Model file for the job. Use its own axes, mm. A direction names the side the tool comes from. Give positions to 0.01 mm unless a question says otherwise; leave off trailing zeros. Write each loop counter-clockwise with the first axis right and the second up, starting at its lowest first coordinate (ties: lowest second). Pieces come first, ordered by that corner, then holes. Notation, with made-up numbers: (-36, 86) - (-29, 86) arc R12 ccw to (-29, 100) - close; hole circle Ø6 at (46, 66.25). An arc over 180 degrees is marked (long way). Use a Markdown table: item, result. Add a question column.
```python
from build123d import *

# Parameters (mm, degrees)
F0_W      = 29
F0_H      = 16.5
F1_DEPTH  = 38.5
F2_SIZE   = 2
F3_SIZE   = 2
F4_SIZE   = 1
F5_W      = 25
F5_H      = 12.5
F6_DEPTH  = 34.25
F8_DEPTH  = 16.501
F9_W      = 12.5
F9_H      = 1
F10_DEPTH = 25
F11_W     = 7.54
F11_H     = 7.25
F11_R     = 1.1
F12_DEPTH = 4.35
F13_R     = 2
F14_DEPTH = 25
F15_W     = 5.538
F15_H     = 5.533
F17_W     = 5.538
F17_H     = 4.538


with BuildPart() as f1:
    # F0 (on Top) → F1 (new body)
    with BuildSketch(Plane.XY):
        with Locations((14.5, 8.25)):
            Rectangle(F0_W, F0_H)
    extrude(amount=F1_DEPTH)

    # F2
    f2_edges = [f1.edges().sort_by_distance(p)[0] for p in [
        (0, 0, 19.25),
        (0, 16.5, 19.25),
        (29, 0, 19.25),
        (29, 16.5, 19.25),
    ]]
    chamfer(f2_edges, length=F2_SIZE)

    # F3
    f3_edges = [f1.edges().sort_by_distance(p)[0] for p in [
        (0, 8.25, 0),
        (1, 15.5, 0),
        (1, 1, 0),
        (14.5, 16.5, 0),
        (14.5, 0, 0),
        (28, 15.5, 0),
        (28, 1, 0),
        (29, 8.25, 0),
    ]]
    chamfer(f3_edges, length=F3_SIZE)

    # F4
    f4_edges = [f1.edges().sort_by_distance(p)[0] for p in [
        (0, 8.25, 38.5),
        (1, 15.5, 38.5),
        (1, 1, 38.5),
        (14.5, 16.5, 38.5),
        (14.5, 0, 38.5),
        (28, 15.5, 38.5),
        (28, 1, 38.5),
        (29, 8.25, 38.5),
    ]]
    chamfer(f4_edges, length=F4_SIZE)

    # F5 (on face) → F6 (cut)
    with BuildSketch(Plane.XY.offset(38.5)):
        with Locations((14.5, 8.25)):
            Rectangle(F5_W, F5_H)
    extrude(amount=-F6_DEPTH, mode=Mode.SUBTRACT)

    # F7 (on face) → F8 (cut, through all)
    with BuildSketch(Plane.XZ):
        Polygon((5.464, 8.664), (5.464, 4.94), (22.536, 4.94), (22.536, 8.664), (16.364, 12.836), (11.636, 12.836), align=None)
    extrude(amount=-F8_DEPTH, mode=Mode.SUBTRACT)

    # F9 (on face) → F10 (cut)
    with BuildSketch(Plane.YZ.offset(29)):
        with BuildLine():
            ThreePointArc((5.0538961688, 23.1590909091), (8.2204306945, 19.7509741882), (11.55, 23))
            ThreePointArc((11.55, 23), (11.5490258118, 23.0795693055), (11.5461038312, 23.1590909091))
            ThreePointArc((11.5461038312, 23.1590909091), (8.3, 22.25), (5.0538961688, 23.1590909091))
        make_face()
        with BuildLine():
            ThreePointArc((5.0538961688, 23.1590909091), (8.3, 22.25), (11.5461038312, 23.1590909091))
            ThreePointArc((11.5461038312, 23.1590909091), (8.3, 26.25), (5.0538961688, 23.1590909091))
        make_face()
        with BuildLine():
            ThreePointArc((5.0538961688, 23.1590909091), (8.3, 26.25), (11.5461038312, 23.1590909091))
            ThreePointArc((11.5461038312, 23.1590909091), (13.5428254576, 25.0977535038), (14.5, 27.7110133081))
            Line((14.5, 27.7110133081), (14.5, 28.5))
            Line((14.5, 28.5), (2.05, 28.5))
            ThreePointArc((2.05, 28.5), (2.8524937382, 25.4361502113), (5.0538961688, 23.1590909091))
        make_face()
        with BuildLine():
            Line((2, 28.5), (2.05, 28.5))
            ThreePointArc((2.05, 28.5), (7.9047152925, 34.7374874749), (14.5, 29.2889866919))
            Line((14.5, 29.2889866919), (14.5, 37.5))
            Line((14.5, 37.5), (2, 37.5))
            Line((2, 37.5), (2, 28.5))
        make_face()
        with BuildLine():
            ThreePointArc((14.5, 29.2889866919), (7.9047152925, 34.7374874749), (2.05, 28.5))
            Line((2.05, 28.5), (14.5, 28.5))
            Line((14.5, 28.5), (14.5, 29.2889866919))
        make_face()
        with Locations((8.25, 38)):
            Rectangle(F9_W, F9_H)
    extrude(amount=-F10_DEPTH, mode=Mode.SUBTRACT)

    # F11 (on face) → F12 (join)
    with BuildSketch(Plane(origin=(0, 0, 0), x_dir=(0, -1, 0), z_dir=(-1, 0, 0))):
        with Locations((-8.25, 7.875)):
            Rectangle(F11_W, F11_H)
        with Locations((-8.25, 9)):
            Circle(F11_R, mode=Mode.SUBTRACT)
    extrude(amount=-F12_DEPTH)

    # F13 (on face) → F14 (cut)
    with BuildSketch(Plane.YZ.offset(2)):
        with Locations((8.25, 22.9216944426)):
            Circle(F13_R)
    extrude(amount=-F14_DEPTH, mode=Mode.SUBTRACT)

    # F15 (on face) → F18 section 0
    with BuildSketch(Plane.YZ.offset(29)):
        with Locations((8.25, 8.0385)):
            Rectangle(F15_W, F15_H)
    # F17 (on offset) → F18 section 1
    with BuildSketch(Plane.YZ.offset(24.55)):
        with Locations((8.25, 8.491)):
            Rectangle(F17_W, F17_H)
    loft(mode=Mode.SUBTRACT)


solid = f1.part
```
(1) Probe probe 1 along Y at (x, z) = (12.75, 33.5); probe 2 along Z at (x, y) = (3.4, 8.25); probe 3 along X at (y, z) = (5, 20). List the from-to ranges inside material, lowest first. Write a range as [from, to].
(2) Which spindle directions (+Z, -Z, +X, -X, +Y, -Y) get a long thin tool onto all of the face, cutting with end or side? Do faces 1 (the cylindrical face through (3.159, 7.234, 8.579)), 2 (the flat face through (14, 16, 38)), 3 (the cylindrical face through (28.01, 2.83, 25.48)), 4 (the flat face through (14, 15, 4.94)). Say none if no direction does.
(3) Band-saw the part on D-D (z = 32). Write the cut outline in (x, y), then the cut area to 3 significant figures.
(4) Band-saw the part on C-C (y = 7.75). Write the cut outline in (x, z) (3 decimals).
(5) Flat gauge pins, fed straight in: pin 1 (1.9 mm diameter, centred on x = 3, y = 9, fed in from +Z); pin 2 (1.6 mm diameter, centred on x = 13.5, y = 1, fed in from -Z); pin 3 (6 mm diameter, centred on y = 7.5, z = 23, fed in from +X); pin 4 (0.6 mm diameter, centred on y = 16, z = 6.5, fed in from -X). Where does each tip first touch, or does it go through?
(6) Two-plate mould, pull along Y, no slides. Class faces 5 (the flat face through (14, 1, 12.836)), 6 (the flat face through (14, 1, 1)), 7 (the flat face through (14, 8, 4.25)), 8 (the flat face through (3, 4.48, 8)): +Y half, -Y half, draft (parallel to the pull), parting line (faces both ways), or undercut.
(7) Band-saw the part on A-A (x = 3.25). Write the cut outline in (y, z), then the cut area to 3 significant figures.
(8) Band-saw the part on B-B (z = 13.5). Write the cut outline in (x, y), then the cut area to 3 significant figures.
Model answer:
| question | item | result |
|---|---|---|
| 1 | probe 1 | y = [0, 2], [14.5, 16.5] |
| 1 | probe 2 | z = [0, 7.9], [10.1, 11.5] |
| 1 | probe 3 | x = [0, 2], [27, 29] |
| 2 | face 1 | +X |
| 2 | face 2 | +Z, +X, -X, +Y |
| 2 | face 3 | +Z, +X |
| 2 | face 4 | +Y, -Y |
| 3 | outline | (0, 2) - (2, 0) - (27, 0) - (29, 2) - (2, 2) - (2, 14.5) - (29, 14.5) - (27, 16.5) - (2, 16.5) - (0, 14.5) - close |
| 3 | area | 133 mm^2 |
| 4 | outline | (0, 2) - (2, 0) - (27, 0) - (29, 2) - (29, 5.272) - (27, 5.699) - (27, 4.25) - (4.35, 4.25) - (4.35, 8.02) - (2, 8.02) - (2, 9.98) - (4.35, 9.98) - (4.35, 11.5) - (2, 11.5) - (2, 20.985) - (0, 20.985) - close; (0, 24.858) - (2, 24.858) - (2, 38.5) - (1, 38.5) - (0, 37.5) - close; (27, 10.785) - (29, 10.805) - (29, 19.797) - (27, 19.797) - close |
| 5 | pin 1 | stops at z = 11.5 |
| 5 | pin 2 | stops at z = 0.2 |
| 5 | pin 3 | stops at x = 29 |
| 5 | pin 4 | stops at x = 1.2 |
| 6 | face 5 | draft |
| 6 | face 6 | -Y half |
| 6 | face 7 | undercut |
| 6 | face 8 | undercut |
| 7 | outline | (0, 2) - (2, 0) - (14.5, 0) - (16.5, 2) - (16.5, 37.5) - (15.5, 38.5) - (14.5, 38.5) - (14.5, 4.25) - (12.02, 4.25) - (12.02, 11.5) - (4.48, 11.5) - (4.48, 4.25) - (2, 4.25) - (2, 38.5) - (1, 38.5) - (0, 37.5) - close; hole circle Ø2.2 at (8.25, 9) |
| 7 | area | 253 mm^2 |
| 8 | outline | (0, 2) - (2, 0) - (27, 0) - (29, 2) - (29, 14.5) - (27, 16.5) - (2, 16.5) - (0, 14.5) - close; hole (2, 2) - (27, 2) - (27, 14.5) - (2, 14.5) - close |
| 8 | area | 158 mm^2 |
